Model file for the job. Use its own axes, mm. Face numbers are marked on the shaded views. Coordinates: 2 decimals unless noted, no trailing zeros. Order: outer loops, then holes, each group sorted by start corner. A loop starts at its lowest first (then second) coordinate and runs counter-clockwise, first axis right, second up.
from build123d import *
from build123d.topology import SkipClean

# Parameters (mm, degrees)
SKETCH1_W            = 42.5
SKETCH1_H            = 24
SKETCH1_R            = 4.5
BOSS_EXTRUDE1_DEPTH  = 2
SKETCH1_2_R          = 4.5
BOSS_EXTRUDE2_DEPTH  = 1
SKETCH2_W            = 1
SKETCH2_H            = 4
FILLET3_START        = -12
FILLET3_DEPTH        = 24
FILLET3_START_2      = -22
FILLET3_2_DEPTH      = 44
FILLET2_R            = 4
M4_CLEARANCE_HOLE1_D = 4.8


with BuildPart() as part:
    # Sketch1 → Boss-Extrude1 (new body)
    with BuildSketch(Plane(origin=(0, 0, 0), x_dir=(1, 0, 0), z_dir=(0, 1, 0))):
        Rectangle(SKETCH1_W, SKETCH1_H)
        with Locations(Location((0, 0, 0), (0, 0, 270))):
            Circle(SKETCH1_R, mode=Mode.SUBTRACT)
        with Locations(Location((16.25, 0, 0), (0, 0, 270))):
            Circle(SKETCH1_R, mode=Mode.SUBTRACT)
        with Locations(Location((-16.25, 0, 0), (0, 0, 270))):
            Circle(SKETCH1_R, mode=Mode.SUBTRACT)
    extrude(amount=BOSS_EXTRUDE1_DEPTH)

    # Sketch1<2> → Boss-Extrude2 (add)
    with BuildSketch(Plane(origin=(0, 0, 0), x_dir=(1, 0, 0), z_dir=(0, 1, 0))):
        with Locations(Location((16.25, 0, 0), (0, 0, 270))):
            Circle(SKETCH1_2_R)
        with Locations(Location((-16.25, 0, 0), (0, 0, 270))):
            Circle(SKETCH1_2_R)
    extrude(amount=BOSS_EXTRUDE2_DEPTH)

    # Sketch2 → Revolve1 (revolve)
    with SkipClean():  # the faces are left unmerged after this step: merging them gives an invalid solid
        with BuildSketch(Plane.XY, mode=Mode.PRIVATE) as revolve1_sk:
            with Locations((-5, 4)):
                Rectangle(SKETCH2_W, SKETCH2_H)
        revolve(revolve1_sk.sketch.rotate(Axis((0, 0, 0), (0, 1, 0)), 270), axis=Axis((0, 0, 0), (0, 1, 0)))
    add(part.part.scale(1), mode=Mode.REPLACE)  # the faces are merged on a copy

    # Fillet3: read off the stored shape, not the designer's step
    # Fillet3 outline → Fillet3 (cut)
    with BuildSketch(Plane.XY.offset(FILLET3_START)):
        with BuildLine():
            Line((21.25, 2), (19.25, 2))
            ThreePointArc((19.25, 2), (20.664213562, 1.414213562), (21.25, 0))
            Line((21.25, 0), (21.25, 2))
        make_face()
        with BuildLine():
            ThreePointArc((-21.25, 0), (-20.664213562, 1.414213562), (-19.25, 2))
            Line((-19.25, 2), (-21.25, 2))
            Line((-21.25, 2), (-21.25, 0))
        make_face()
    extrude(amount=FILLET3_DEPTH, mode=Mode.SUBTRACT)

    # Fillet3 2 outline → Fillet3 2 (cut)
    with BuildSketch(Plane.YZ.offset(FILLET3_START_2)):
        with BuildLine():
            Line((2, -12), (2, -10))
            ThreePointArc((2, -10), (1.414213562, -11.414213562), (0, -12))
            Line((0, -12), (2, -12))
        make_face()
        with BuildLine():
            ThreePointArc((0, 12), (1.414213562, 11.414213562), (2, 10))
            Line((2, 10), (2, 12))
            Line((2, 12), (0, 12))
        make_face()
    extrude(amount=FILLET3_2_DEPTH, mode=Mode.SUBTRACT)

    # Fillet2
    fillet2_edges = [part.edges().sort_by_distance(p)[0] for p in [
        (0, 2, 5.5),
    ]]
    fillet(fillet2_edges, radius=FILLET2_R - 0.0001)  # a hair under: the kernel refuses the full size

    # M4 Clearance Hole1 (through all)
    with Locations(Plane(origin=(0, 0, 0), x_dir=(-1, 0, 0), z_dir=(0, -1, 0))):
        with Locations((-16.25, 0), (16.25, 0)):
            Hole(M4_CLEARANCE_HOLE1_D / 2)


solid = part.part
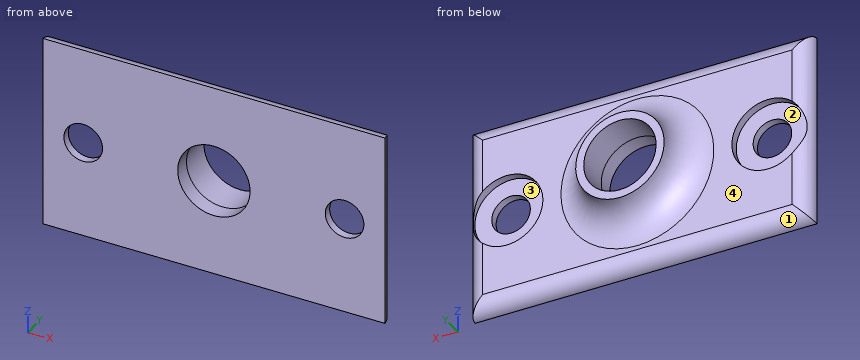
Q1. Cut at A-A, the plane x = 16.25. List the corners of the cut face in (y, z), plus the area to 3 significant figures.
Established:
outline: (0, -12) arc R2 ccw to (2, -10) - (2, -4.5) - (1, -4.5) - (1, -2.4) - (0, -2.4) - close; (0, 2.4) - (1, 2.4) - (1, 4.5) - (2, 4.5) - (2, 10) arc R2 ccw to (0, 12) - close
area: 32.5 mm2
Q2. Cut at B-B, the plane z = 0. Count the separate pieces of the cut face and the enclosed holes in it, plus the area to 3 significant figures.
Established:
separate pieces: 4
enclosed holes: 0
area: 53.2 mm2
Q3. Drop flat-ended pins along their axis: P1, Ø2.5, axis at x = -17.5, z = 2, coming from the +Y side; P2, Ø10, axis at x = 18, z = -2, coming from the +Y side; P3, Ø6, axis at x = 8, z = -6.5, coming from the +Y side. Give the stop position or say it passes through.
Established:
P1: stops at y = 1
P2: stops at y = 2
P3: stops at y = 2.65
Q4. Cut at C-C, the plane y = 0.5. List the corners of the cut face in (x, z), plus the area to 3 significant figures.
Established:
outline: (-21.19, -11.94) - (21.19, -11.94) - (21.19, 11.94) - (-21.19, 11.94) - close; hole circle Ø4.8 at (-16.25, 0); hole circle Ø9 at (0, 0); hole circle Ø4.8 at (16.25, 0)
area: 912 mm2
Q5. Mould opens along Z. For the marked faces 1, 2, 3 and 4 say: pulls with the +Z half, pulls with the -Z half, needs draft (parallel to the pull), parting line crosses it, or undercut.
Established:
face 1: pulls with the -Z half
face 2: undercut
face 3: undercut
face 4: needs draft
Q6. Probe line 1 (X direction, y = 1.75, z = 0); line 2 (Z direction, x = 3, y = 2.5); line 3 (Z direction, x = -0.5, y = 1.75). List the from-to ranges inside material, lowest first.
Established:
line 1: x = -11.75 to -4.5, 4.5 to 11.75
line 2: z = -6.94 to -3.35, 3.35 to 6.94
line 3: z = -10.97 to -4.47, 4.47 to 10.97
